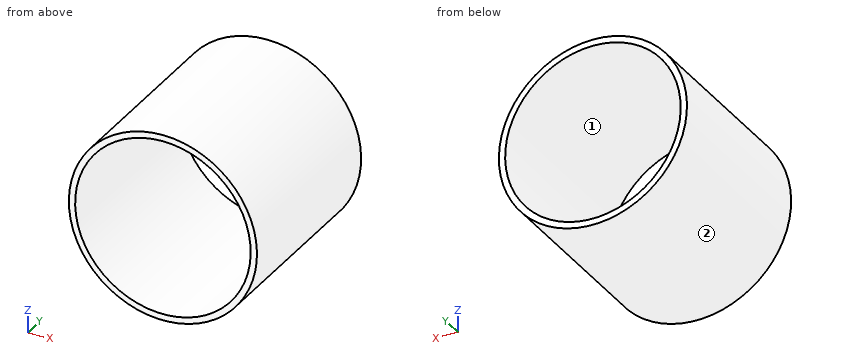
from build123d import *

# Parameters (mm, degrees)
SKETCH1_R               = 75
BOSS_EXTRUDE1_DEPTH     = 75
CUT_EXTRUDE1_DEPTH      = 130.903810568
CUT_EXTRUDE1_DEPTH_BACK = 95
SKETCH2_R               = 70
SKETCH3_R               = 7.5
CUT_EXTRUDE2_DEPTH      = 201.374649095


with BuildPart() as part:
    # Sketch1 → Boss-Extrude1 (new, symmetric)
    with BuildSketch(Plane(origin=(0, 0, 0), x_dir=(1, 0, 0), z_dir=(0, 1, 0))):
        with Locations(Location((0, 0, 0), (0, 0, 270))):
            Circle(SKETCH1_R)
    extrude(amount=BOSS_EXTRUDE1_DEPTH, both=True)

    # Sketch2 → Cut-Extrude1 (cut, two sides: drawn at the far end of the back side and taken through both)
    with BuildSketch(Plane(origin=(0, 0, 0), x_dir=(1, 0, 0), z_dir=(0, 1, 0)).offset(-CUT_EXTRUDE1_DEPTH_BACK)):
        with Locations(Location((0, 0, 0), (0, 0, 270))):
            Circle(SKETCH2_R)
    extrude(amount=CUT_EXTRUDE1_DEPTH + CUT_EXTRUDE1_DEPTH_BACK, mode=Mode.SUBTRACT)

    # Sketch3 → Cut-Extrude2 (cut, through all)
    with BuildSketch(Plane(origin=(0, -95, 0), x_dir=(1, 0, 0), z_dir=(0, 1, 0))):
        Circle(SKETCH3_R)
    extrude(amount=-CUT_EXTRUDE2_DEPTH, mode=Mode.SUBTRACT)


solid = part.part
Check sheet for the modelled part. Datum: model origin and axes. Units: mm. Face numbers are marked on the shaded views. Give positions to 0.01 mm unless a question says otherwise; leave off trailing zeros. Write each loop counter-clockwise with the first axis right and the second up, starting at its lowest first coordinate (ties: lowest second). Pieces come first, ordered by that corner, then holes. Notation, with made-up numbers: (18.25, -35) -> (76.25, -35) arc R18 ccw to (76.25, -17) -> close; hole circle Ø5 at (53.5, 3). An arc over 180 degrees is marked (long way). One line per item, written item: value. Start each with the question number.
Item 1: Material ranges on probe 1 along X at (y, z) = (-19, 0); probe 2 along Z at (x, y) = (16, -17); probe 3 along X at (y, z) = (-52.5, -48), recorded low to high. Write a range as from..to.
Item 2: Section check C-C on y = 18. Record the cut outline in (x, z), then the cut area to 3 significant figures.
Item 3: Section check B-B on z = 0. Record the cut outline in (x, y), then the cut area to 3 significant figures.
Item 4: Draft check along X on the marked faces 1 and 2. Enter one of: +X half, -X half, draft (parallel to the pull), parting line (faces both ways), or undercut.
Item 5: Section check A-A on x = 0. Record the cut outline in (y, z).
Item 6: Gauge pin test, flat ends, axial feed: pin 1 (5 mm diameter, centred on x = 40, y = 14.5, fed in from -Z); pin 2 (3 mm diameter, centred on x = 26.5, y = -55.5, fed in from +Z); pin 3 (6 mm diameter, centred on x = 38, y = -58.5, fed in from +Z). Record the tip position at first contact, or that the pin passes through.
Results list:
1. probe 1: -75..-70, 70..75
1. probe 2: -73.27..-68.15, 68.15..73.27
1. probe 3: -57.63..-50.95, 50.95..57.63
2. outline: circle Ø150 at (0, 0); hole circle Ø140 at (0, 0)
2. area: 2,280 mm²
3. outline: (-75, -75) -> (-70, -75) -> (-70, 75) -> (-75, 75) -> close; (70, -75) -> (75, -75) -> (75, 75) -> (70, 75) -> close
3. area: 1,500 mm²
4. face 1: undercut
4. face 2: parting line
5. outline: (-75, -75) -> (75, -75) -> (75, -70) -> (-75, -70) -> close; (-75, 70) -> (75, 70) -> (75, 75) -> (-75, 75) -> close
6. pin 1: z = -64.95
6. pin 2: z = 70.71
6. pin 3: z = 66.33
